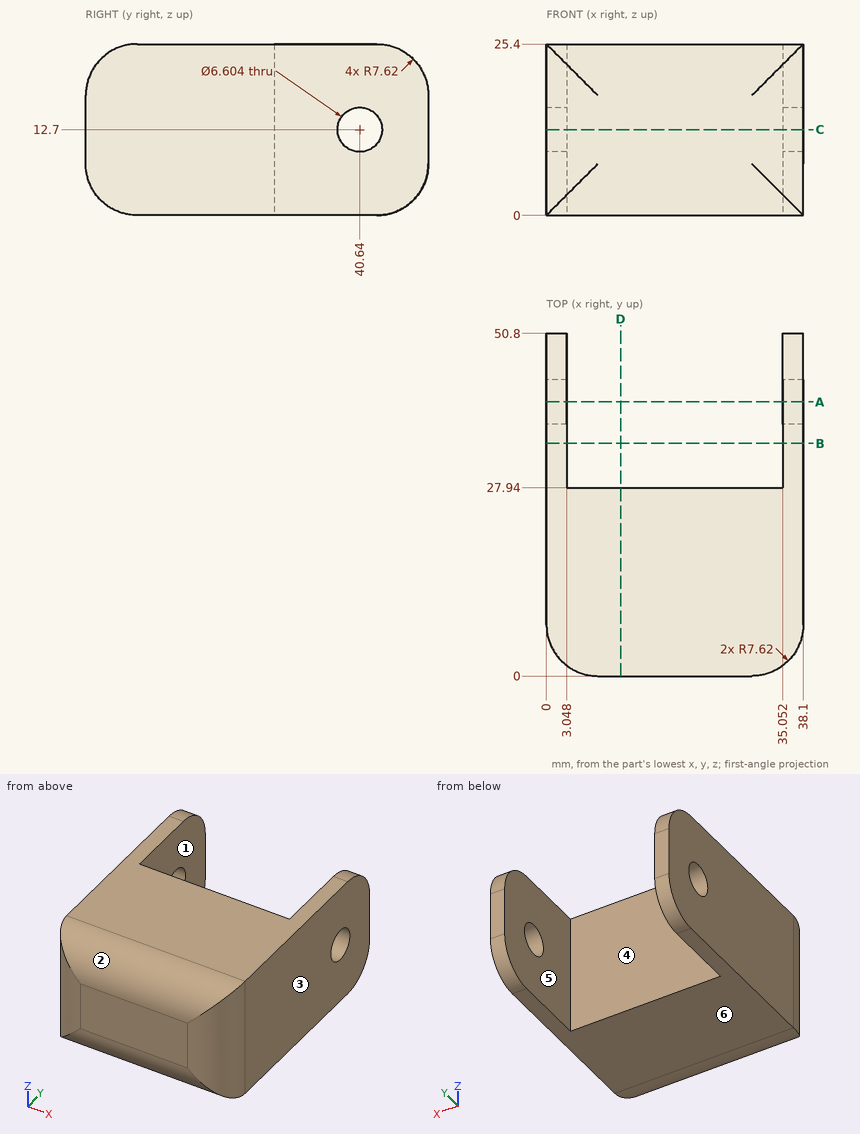
Part print with two shaded views. Sizes in mm from the minimum x, y, z corner. A direction names the side the tool comes from. Give positions to 0.01 mm unless a question says otherwise; leave off trailing zeros. Order: outer loops, then holes, each group sorted by start corner. A loop starts at its lowest first (then second) coordinate and runs counter-clockwise, first axis right, second up.
(1) Saw through at A-A, the plane y = 40.64. Give the cut face in (x, z), then the cut area to 3 significant figures.
(2) Tool access for the marked faces 5 and 6: list every direction of +Z, -Z, +X, -X, +Y, -Y with a clear straight run to the whole face (end or side of a thin tool).
(3) Saw through at B-B, the plane y = 34.5. Give the cut face in (x, z), then the cut area to 3 significant figures.
(4) Saw through at D-D, the plane x = 11. Give the cut face in (y, z).
(5) Drill centre lines: L1, parallel to X at y = 39.5, z = 16; L2, parallel to Y at x = 0.7, z = 12.7; L3, parallel to Y at x = 1.5, z = 12.7. Where is each one in solid material? Low to high.
(6) Flat gauge pins, fed straight in: pin 1 (5 mm diameter, centred on x = 30.5, z = 12.5, fed in from +Y); pin 2 (5.5 mm diameter, centred on y = 40.64, z = 12.7, fed in from -X). Where does each tip first touch, or does it go through?
(7) Mould opens along X. For the marked faces 1, 2, 3 and 4 say: released by +X, released by -X, zero draft, split by the parting line, or undercut.
(8) Saw through at C-C, the plane z = 12.7. Give the cut face in (x, y), then the cut area to 3 significant figures.
Results found:
1. outline: (0, 0) - (3.05, 0) - (3.05, 9.4) - (0, 9.4) - close; (0, 16) - (3.05, 16) - (3.05, 25.4) - (0, 25.4) - close; (35.05, 0) - (38.1, 0) - (38.1, 9.4) - (35.05, 9.4) - close; (35.05, 16) - (38.1, 16) - (38.1, 25.4) - (35.05, 25.4) - close
1. area: 115 mm2
2. face 5: +Z, -Z, +Y
2. face 6: -Z, +X, -X, +Y, -Y
3. outline: (0, 0) - (3.05, 0) - (3.05, 25.4) - (0, 25.4) - close; (35.05, 0) - (38.1, 0) - (38.1, 25.4) - (35.05, 25.4) - close
3. area: 155 mm2
4. outline: (0, 7.62) arc R7.62 ccw to (7.62, 0) - (27.94, 0) - (27.94, 25.4) - (7.62, 25.4) arc R7.62 ccw to (0, 17.78) - close
5. L1: x = 0 to 3.05, 35.05 to 38.1
5. L2: y = 4.43 to 37.34, 43.94 to 50.8
5. L3: y = 3.08 to 37.34, 43.94 to 50.8
6. pin 1: stops at y = 27.94
6. pin 2: passes through
7. face 1: undercut
7. face 2: zero draft
7. face 3: released by +X
7. face 4: undercut
8. outline: (0, 7.62) arc R7.62 ccw to (7.62, 0) - (30.48, 0) arc R7.62 ccw to (38.1, 7.62) - (38.1, 37.34) - (35.05, 37.34) - (35.05, 27.94) - (3.05, 27.94) - (3.05, 37.34) - (0, 37.34) - close; (0, 43.94) - (3.05, 43.94) - (3.05, 50.8) - (0, 50.8) - close; (35.05, 43.94) - (38.1, 43.94) - (38.1, 50.8) - (35.05, 50.8) - close
8. area: 1,140 mm2
